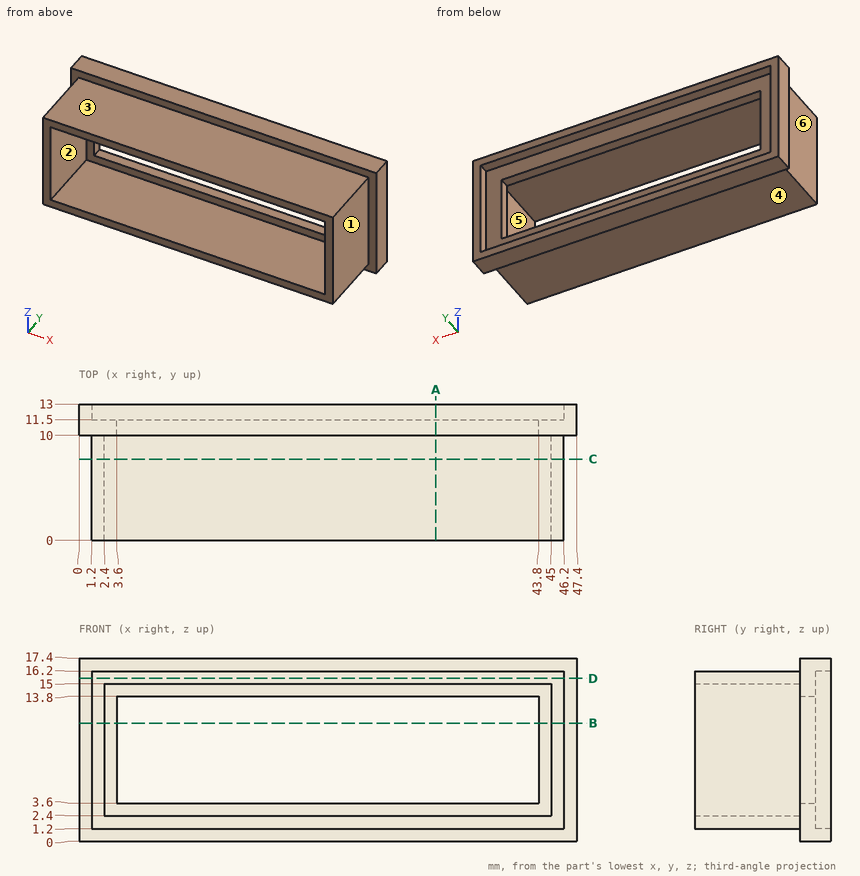
Could you check a few things on this drawing? It's one solid part, dimensions in mm from its lowest x, y, z. A direction names the side the tool comes from. Round coordinates to 2 decimals unless told otherwise and drop trailing zeros. Write each loop counter-clockwise with the first axis right and the second up, starting at its lowest first coordinate (ties: lowest second). Pieces come first, ordered by that corner, then holes. Notation, with made-up numbers: (79.5, 85) -> (135.5, 85) arc R19 cw to (135.5, 120) -> close; hole circle Ø11 at (-34, 70.5). An arc over 180 degrees is marked (long way). One line per item, written item: value.
1) Suppose I cut it at C-C on y = 7.75. List the corners of the cut face in (x, z) for me.
Filled sheet:
outline: (1.2, 1.2) -> (46.2, 1.2) -> (46.2, 16.2) -> (1.2, 16.2) -> close; hole (2.4, 2.4) -> (45, 2.4) -> (45, 15) -> (2.4, 15) -> close
2) I'm going to push flat-ended pins straight in: pin 1 Ø5 at (y, z) = (2, 5) entering from -X; pin 2 Ø5 at (x, y) = (31.5, 4) entering from -Z; pin 3 Ø3 at (x, y) = (21.5, 5.5) entering from +Z. Where does each tip first touch, or does it pass through?
Filled sheet:
pin 1: stops at x = 1.2
pin 2: stops at z = 1.2
pin 3: stops at z = 16.2
3) Suppose I cut it at D-D on z = 15.5. List the corners of the cut face in (x, y) for me, plus the area to 3 significant figures.
Filled sheet:
outline: (0, 10) -> (1.2, 10) -> (1.2, 0) -> (46.2, 0) -> (46.2, 10) -> (47.4, 10) -> (47.4, 13) -> (46.2, 13) -> (46.2, 11.5) -> (1.2, 11.5) -> (1.2, 13) -> (0, 13) -> close
area: 525 mm2
4) We'd pull the mould along Z, two halves only. Please class the marked faces 1, 2 and 3: released by +Z, released by -Z, zero draft, split by the parting line, or undercut.
Filled sheet:
face 1: zero draft
face 2: undercut
face 3: released by +Z
5) Suppose I cut it at B-B on z = 11.25. List the corners of the cut face in (x, y) for me, plus the area to 3 significant figures.
Filled sheet:
outline: (0, 10) -> (1.2, 10) -> (1.2, 0) -> (2.4, 0) -> (2.4, 10) -> (3.6, 10) -> (3.6, 11.5) -> (1.2, 11.5) -> (1.2, 13) -> (0, 13) -> close; (43.8, 10) -> (45, 10) -> (45, 0) -> (46.2, 0) -> (46.2, 10) -> (47.4, 10) -> (47.4, 13) -> (46.2, 13) -> (46.2, 11.5) -> (43.8, 11.5) -> close
area: 38.4 mm2
6) Suppose I cut it at A-A on x = 34. List the corners of the cut face in (y, z) for me.
Filled sheet:
outline: (0, 1.2) -> (10, 1.2) -> (10, 0) -> (13, 0) -> (13, 1.2) -> (11.5, 1.2) -> (11.5, 3.6) -> (10, 3.6) -> (10, 2.4) -> (0, 2.4) -> close; (0, 15) -> (10, 15) -> (10, 13.8) -> (11.5, 13.8) -> (11.5, 16.2) -> (13, 16.2) -> (13, 17.4) -> (10, 17.4) -> (10, 16.2) -> (0, 16.2) -> close
7) If I drill on line 1 (Z direction, x = 41, y = 5.25); line 2 (Z direction, x = 31.5, y = 12); line 3 (X direction, y = 11.75, z = 9), over which ranges is the centre line in solid material (lowest first)? Write a range as [from, to].
Filled sheet:
line 1: z = [1.2, 2.4], [15, 16.2]
line 2: z = [0, 1.2], [16.2, 17.4]
line 3: x = [0, 1.2], [46.2, 47.4]
8) For the marked faces 4, 5 and 6, which set-ups out of +Z, -Z, +X, -X, +Y, -Y let a thin tool reach every point of the face, with its end or its side?
Filled sheet:
face 4: -Z, +X, -X, -Y
face 5: -Y
face 6: +Z, -Z, -X, -Y
